Drawing for the job (mm, zero at the part's lowest x, y, z). A direction names the side the tool comes from. Round coordinates to 2 decimals unless told otherwise and drop trailing zeros. Write each loop counter-clockwise with the first axis right and the second up, starting at its lowest first coordinate (ties: lowest second). Pieces come first, ordered by that corner, then holes. Notation, with made-up numbers: (11.5, 68) - (62.5, 68) arc R26 ccw to (62.5, 100) - close; hole circle Ø4 at (5.25, 13.25). An arc over 180 degrees is marked (long way). Answer in a Markdown table with one row per item.
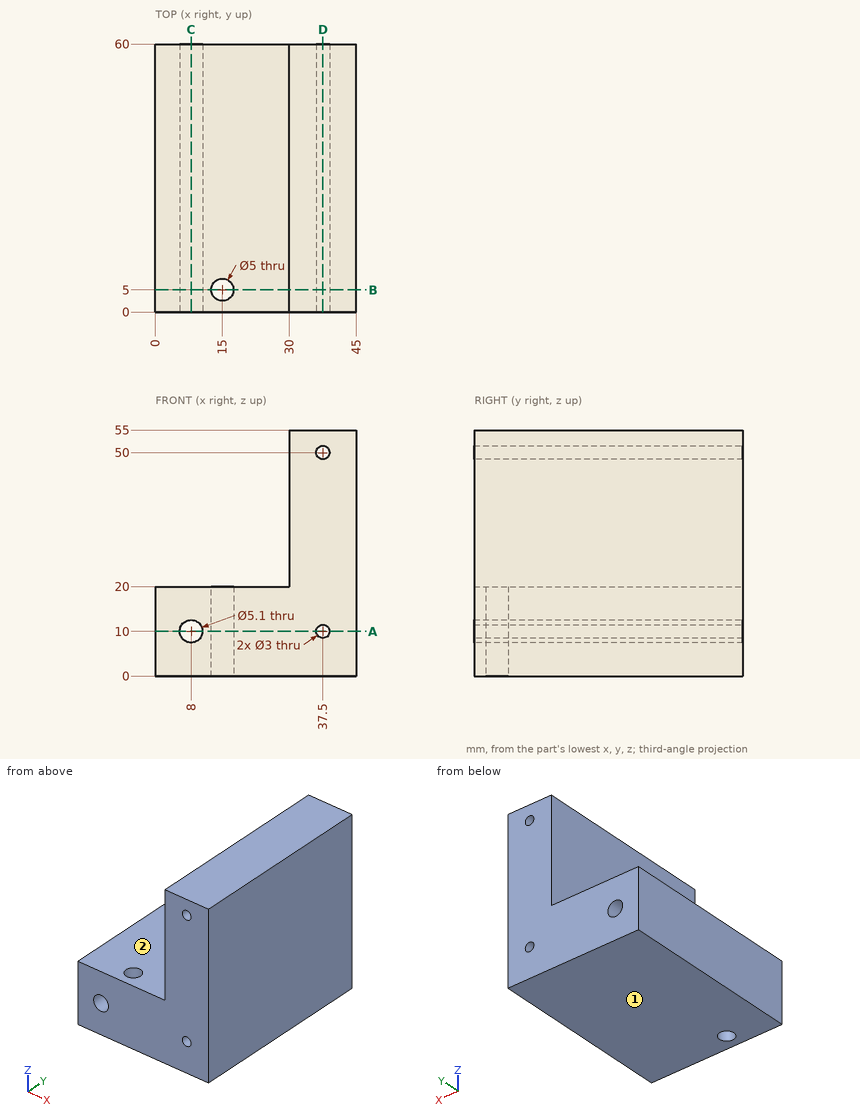
Q1. Saw through at D-D on x = 37.5. List the corners of the cut face in (y, z), then the cut area to 3 significant figures.
Computed:
| item | result |
|---|---|
| outline | (0, 0) - (60, 0) - (60, 8.5) - (0, 8.5) - close; (0, 11.5) - (60, 11.5) - (60, 48.5) - (0, 48.5) - close; (0, 51.5) - (60, 51.5) - (60, 55) - (0, 55) - close |
| area | 2,940 mm2 |
Q2. Saw through at C-C on x = 8. List the corners of the cut face in (y, z).
Computed:
| item | result |
|---|---|
| outline | (0, 0) - (60, 0) - (60, 7.45) - (0, 7.45) - close; (0, 12.55) - (60, 12.55) - (60, 20) - (0, 20) - close |
Q3. Saw through at A-A on z = 10. List the corners of the cut face in (x, y).
Computed:
| item | result |
|---|---|
| outline | (0, 0) - (5.45, 0) - (5.45, 60) - (0, 60) - close; (10.55, 0) - (36, 0) - (36, 60) - (10.55, 60) - close; (39, 0) - (45, 0) - (45, 60) - (39, 60) - close; hole circle Ø5 at (15, 5) |
Q4. Saw through at B-B on y = 5. List the corners of the cut face in (x, z).
Computed:
| item | result |
|---|---|
| outline | (0, 0) - (12.5, 0) - (12.5, 20) - (0, 20) - close; (17.5, 0) - (45, 0) - (45, 55) - (30, 55) - (30, 20) - (17.5, 20) - close; hole circle Ø5.1 at (8, 10); hole circle Ø3 at (37.5, 10); hole circle Ø3 at (37.5, 50) |
Q5. 3-axis set-ups, long thin cutter, end or side, ignore diameter. For the marked faces 1 and 2: which of +Z, -Z, +X, -X, +Y, -Y reach the whole face in a straight line?
Computed:
| item | result |
|---|---|
| face 1 | -Z, +X, -X, +Y, -Y |
| face 2 | +Z, -X, +Y, -Y |
Q6. Drill centre lines: line 1 (Y direction, x = 15, z = 15); line 2 (X direction, y = 17, z = 50); line 3 (Z direction, x = 37, y = 12). Where is each one in solid material? Low to high.
Computed:
| item | result |
|---|---|
| line 1 | y = 0 to 2.5, 7.5 to 60 |
| line 2 | x = 30 to 36, 39 to 45 |
| line 3 | z = 0 to 8.59, 11.41 to 48.59, 51.41 to 55 |
Q7. Flat gauge pins, fed straight in: pin 1 (3 mm diameter, centred on y = 41.5, z = 36.5, fed in from -X); pin 2 (3 mm diameter, centred on x = 28, y = 18.5, fed in from +Z). Where does each tip first touch, or does it go through?
Computed:
| item | result |
|---|---|
| pin 1 | stops at x = 30 |
| pin 2 | stops at z = 20 |
